from build123d import *

# Parameters (mm, degrees)
ESQUISSE1_R             = 25
ESQUISSE1_R_2           = 1.7
BOSS_EXTRU_1_DEPTH      = 3
ESQUISSE6_R             = 11
ENL_V_MAT_EXTRU_2_DEPTH = 36.482389998
BOSS_EXTRU_6_DEPTH      = 3
ESQUISSE11_W            = 18.64617436
ESQUISSE11_H            = 6
ENL_V_MAT_EXTRU_3_DEPTH = 36.482389998
ESQUISSE12_W            = 17.120822442
ESQUISSE12_H            = 1.5
ESQUISSE13_W            = 17.212222589
ESQUISSE13_H            = 1.5
ESQUISSE14_W            = 6.427132246
ESQUISSE14_H            = 29.186840833
ENL_V_MAT_EXTRU_4_DEPTH = 36.482390148


with BuildPart() as part:
    # Esquisse1 → Boss.-Extru.1 (new body)
    with BuildSketch(Plane.XY):
        Circle(ESQUISSE1_R)
        with Locations((-13.435028843, 13.435028843)):
            Circle(ESQUISSE1_R_2, mode=Mode.SUBTRACT)
        with Locations((13.435028843, 13.435028843)):
            Circle(ESQUISSE1_R_2, mode=Mode.SUBTRACT)
        with Locations((13.435028843, -13.435028843)):
            Circle(ESQUISSE1_R_2, mode=Mode.SUBTRACT)
        with Locations((-13.435028843, -13.435028843)):
            Circle(ESQUISSE1_R_2, mode=Mode.SUBTRACT)
    extrude(amount=BOSS_EXTRU_1_DEPTH)

    # Esquisse6 → Enlèv. mat.-Extru.2 (cut, through all)
    with BuildSketch(Plane(origin=(0, 0, 0), x_dir=(-1, 0, 0), z_dir=(0, 0, -1))):
        Circle(ESQUISSE6_R)
    extrude(amount=-ENL_V_MAT_EXTRU_2_DEPTH, mode=Mode.SUBTRACT)

    # Esquisse10 → Boss.-Extru.6 (add)
    with BuildSketch(Plane.XY.offset(3)):
        with BuildLine():
            Line((-5.758802096, -2.316766812), (-9.508802096, -5.566766812))
            ThreePointArc((-9.508802096, -5.566766812), (-10.566766812, -5.491197904), (-10.491197904, -4.433233188))
            Line((-10.491197904, -4.433233188), (-6.741197904, -1.183233188))
            ThreePointArc((-6.741197904, -1.183233188), (-5.683233188, -1.258802096), (-5.758802096, -2.316766812))
        make_face()
        with BuildLine():
            Line((-6.741197904, 1.183233188), (-10.491197904, 4.433233188))
            ThreePointArc((-10.491197904, 4.433233188), (-10.566766812, 5.491197904), (-9.508802096, 5.566766812))
            Line((-9.508802096, 5.566766812), (-5.758802096, 2.316766812))
            ThreePointArc((-5.758802096, 2.316766812), (-5.683233188, 1.258802096), (-6.741197904, 1.183233188))
        make_face()
        with BuildLine():
            Line((9.508802096, -5.566766812), (5.758802096, -2.316766812))
            ThreePointArc((5.758802096, -2.316766812), (5.683233188, -1.258802096), (6.741197904, -1.183233188))
            Line((6.741197904, -1.183233188), (10.491197904, -4.433233188))
            ThreePointArc((10.491197904, -4.433233188), (10.566766812, -5.491197904), (9.508802096, -5.566766812))
        make_face()
        with BuildLine():
            Line((10.491197904, 4.433233188), (6.741197904, 1.183233188))
            ThreePointArc((6.741197904, 1.183233188), (5.683233188, 1.258802096), (5.758802096, 2.316766812))
            Line((5.758802096, 2.316766812), (9.508802096, 5.566766812))
            ThreePointArc((9.508802096, 5.566766812), (10.566766812, 5.491197904), (10.491197904, 4.433233188))
        make_face()
    extrude(amount=-BOSS_EXTRU_6_DEPTH)

    # Esquisse11 → Enlèv. mat.-Extru.3 (cut, through all)
    with BuildSketch(Plane.XY.offset(3)):
        with Locations((-19.368578738, 0)):
            Rectangle(ESQUISSE11_W, ESQUISSE11_H)
    extrude(amount=-ENL_V_MAT_EXTRU_3_DEPTH, mode=Mode.SUBTRACT)

    # Esquisse12 → Enlèvement de matière-Révolution1 (revolve, cut)
    with BuildSketch(Plane.XY.offset(3)):
        with Locations((-15.814736021, -6.304475395)):
            Rectangle(ESQUISSE12_W, ESQUISSE12_H)
    revolve(axis=Axis((-24.375147242, -7.054475395, 3), (1, 0, 0)), mode=Mode.SUBTRACT)

    # Esquisse13 → Enlèvement de matière-Révolution2 (revolve, cut)
    with BuildSketch(Plane.XY.offset(3)):
        with Locations((-15.769035948, 6.304475395)):
            Rectangle(ESQUISSE13_W, ESQUISSE13_H)
    revolve(axis=Axis((-24.375147242, 7.054475395, 3), (1, 0, 0)), mode=Mode.SUBTRACT)

    # Esquisse14 → Enlèv. mat.-Extru.4 (cut, through all)
    with BuildSketch(Plane.XY.offset(3)):
        with Locations((24.296734765, 1.158391573)):
            Rectangle(ESQUISSE14_W, ESQUISSE14_H)
    extrude(amount=-ENL_V_MAT_EXTRU_4_DEPTH, mode=Mode.SUBTRACT)


solid = part.part
The listing builds one solid part. Answer for the finished solid, in the listing's coordinates (mm). A direction names the side the tool comes from. Coordinates: 2 decimals unless noted, no trailing zeros. Order: outer loops, then holes, each group sorted by start corner. A loop starts at its lowest first (then second) coordinate and runs counter-clockwise, first axis right, second up. Notation, with made-up numbers: (47, 42) -> (95, 42) arc R19 cw to (95, 58) -> close; hole circle Ø1 at (14.25, 68). An arc over 180 degrees is marked (long way). Answer in a Markdown table with one row per item. Add a question column.
Item 1: Which of the six approach directions +Z, -Z, +X, -X, +Y, -Y give full straight-line access (tool end or side, diameter ignored) to faces 4 (the face through (-18, -3, 2)), 5 (the face through (-7.7, 4, 1.5)), 6 (the face through (4, -11, 0)), 7 (the face through (-15.6, 7, 1.5))?
Item 2: Find section A-A (z = 0.9). Write down the section's boundary in (x, y).
Item 3: Find section C-C (x = 7.5). Write down the section's boundary in (y, z).
Item 4: Determine the mould class of faces 1 (the face through (4, -11, 3)), 2 (the face through (-5.96, -24.28, 1.48)), 3 (the face through (5.673, -1.271, 1.521)) for opening direction Y: +Y half, -Y half, draft (parallel to the pull), parting line (faces both ways), or undercut.
Item 5: Each of these flat-tipped pins is pushed along its axis until it touches: P1, Ø0.9, axis at x = -18.5, z = 1, coming from the -Y side; P2, Ø0.9, axis at x = -15.5, z = 1, coming from the +Y side; P3, Ø3, axis at x = -13.44, y = -13.44, coming from the +Z side; P4, Ø1.5, axis at y = 6, z = 1, coming from the -X side. Where does it stop, or does it pass through?
Item 6: Find section B-B (y = 14). Write down the section's boundary in (x, z), then the cut area to 3 significant figures.
Item 7: Find section D-D (x = 1.5). Write down the section's boundary in (y, z), then the cut area to 3 significant figures.
Item 8: Find the intervals of material crossed by L1, parallel to Y at x = -17, z = 2.85; L2, parallel to X at y = -3.5, z = 0.2; L3, parallel to Y at x = -12.5, z = 1.9, in increasing order. Write a range as from..to.
Result set:
| question | item | result |
|---|---|---|
| 1 | face 4 | +Z, -Z, -X |
| 1 | face 5 | +Z, -Z |
| 1 | face 6 | -Z, +X, -X, +Y, -Y |
| 1 | face 7 | +Z, -X |
| 2 | outline | (-24.82, -3) arc R25 ccw to (21.08, -13.44) -> (21.08, 13.44) arc R25 ccw to (-24.82, 3) -> (-10.58, 3) arc R11 cw to (-10.18, 4.16) -> (-6.74, 1.18) arc R0.75 ccw to (-5.76, 2.32) -> (-9.49, 5.55) arc R11 cw to (9.49, 5.55) -> (5.76, 2.32) arc R0.75 ccw to (6.74, 1.18) -> (10.18, 4.16) arc R11 cw to (10.18, -4.16) -> (6.74, -1.18) arc R0.75 ccw to (5.76, -2.32) -> (9.49, -5.55) arc R11 cw to (-9.49, -5.55) -> (-5.76, -2.32) arc R0.75 ccw to (-6.74, -1.18) -> (-10.18, -4.16) arc R11 cw to (-10.58, -3) -> close; hole circle Ø3.4 at (-13.44, -13.44); hole circle Ø3.4 at (-13.44, 13.44); hole circle Ø3.4 at (13.44, -13.44); hole circle Ø3.4 at (13.44, 13.44) |
| 3 | outline | (-23.85, 0) -> (-8.05, 0) -> (-8.05, 3) -> (-23.85, 3) -> close; (-3.83, 0) -> (-1.84, 0) -> (-1.84, 3) -> (-3.83, 3) -> close; (1.84, 0) -> (3.83, 0) -> (3.83, 3) -> (1.84, 3) -> close; (8.05, 0) -> (23.85, 0) -> (23.85, 3) -> (8.05, 3) -> close |
| 4 | face 1 | draft |
| 4 | face 2 | -Y half |
| 4 | face 3 | undercut |
| 5 | P1 | stops at y = -17.3 |
| 5 | P2 | stops at y = 19.96 |
| 5 | P3 | passes through |
| 5 | P4 | stops at x = -24.44 |
| 6 | outline | (-20.71, 0) -> (-15.04, 0) -> (-15.04, 3) -> (-20.71, 3) -> close; (-11.83, 0) -> (11.83, 0) -> (11.83, 3) -> (-11.83, 3) -> close; (15.04, 0) -> (20.71, 0) -> (20.71, 3) -> (15.04, 3) -> close |
| 6 | area | 105 mm² |
| 7 | outline | (-24.95, 0) -> (-10.9, 0) -> (-10.9, 3) -> (-24.95, 3) -> close; (10.9, 0) -> (24.95, 0) -> (24.95, 3) -> (10.9, 3) -> close |
| 7 | area | 84.3 mm² |
| 8 | L1 | y = -18.33..-8.55, -5.56..-3, 3..5.56, 8.55..18.33 |
| 8 | L2 | x = -24.75..-10.43, -9.41..-7.12, 7.12..9.41, 10.43..21.08 |
| 8 | L3 | y = -21.65..-14.85, -12.02..-8.07, -6.03..-3, 3..6.03, 8.07..12.02, 14.85..21.65 |
